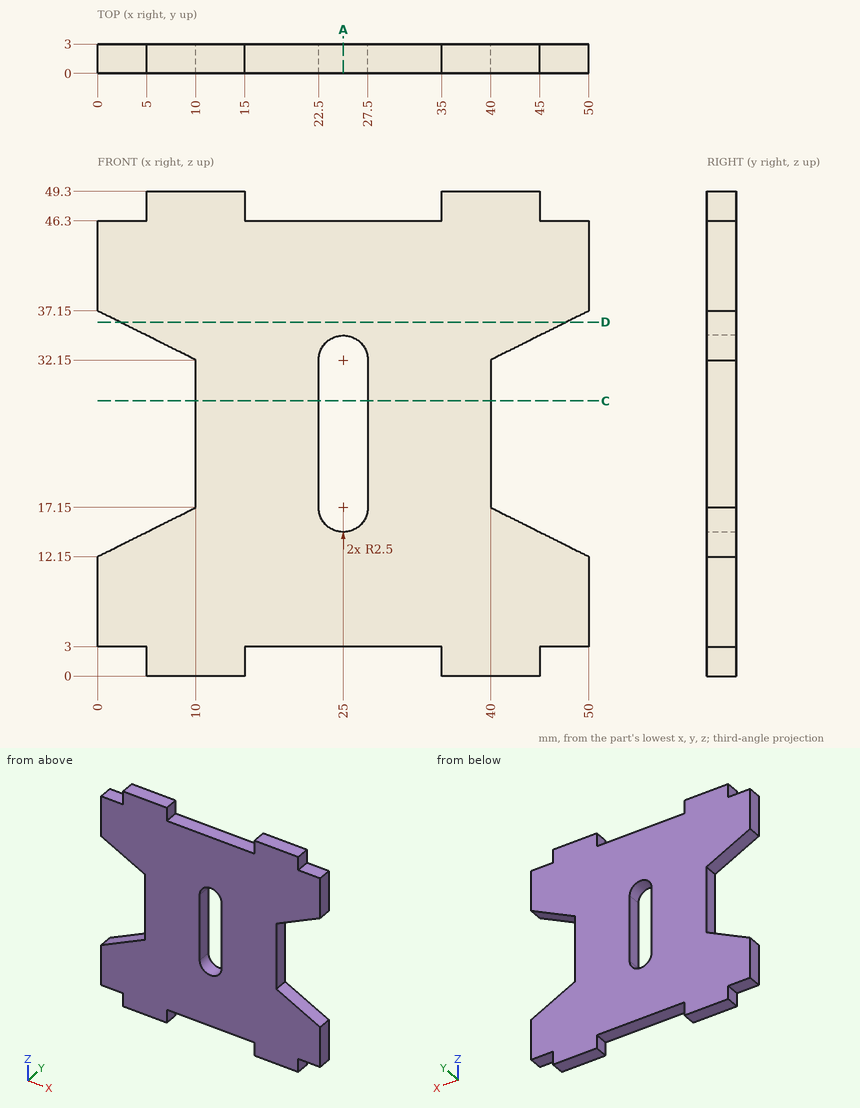
Drawing for the job (mm, zero at the part's lowest x, y, z). Coordinates: 2 decimals unless noted, no trailing zeros. Loops run counter-clockwise (first coordinate to the right, second up) from the corner with the lowest first, then second, coordinate; pieces in that order, holes last. Notation, with made-up numbers: (-9.5, 2.5) - (27.5, 2.5) arc R19 ccw to (27.5, 26.5) - close; hole circle Ø3 at (12, 84.5). An arc over 180 degrees is marked (long way). Use CSV: the item, a comma, the result in double quotes. Start each with the question number.
Q1. Cut at D-D, the plane z = 36. List the corners of the cut face in (x, y), then the cut area to 3 significant figures.
Q2. Probe probe 1 along X at (y, z) = (0.35, 27); probe 2 along Z at (x, y) = (29, 1.5); probe 3 along Z at (x, y) = (2.5, 1.5). List the from-to ranges inside material, lowest first. Write a range as from..to.
Q3. Cut at A-A, the plane x = 25. List the corners of the cut face in (y, z), then the cut area to 3 significant figures.
Q4. Drop flat-ended pins along their axis: P1, Ø0.9, axis at x = 2, y = 1, coming from the -Z side; P2, Ø1.5, axis at y = 2, z = 28, coming from the -X side; P3, Ø0.9, axis at y = 1.5, z = 2, coming from the -X side. Give the stop position or say it passes through.
Q5. Cut at C-C, the plane z = 28. List the corners of the cut face in (x, y), then the cut area to 3 significant figures.
Here are the results:
1,outline,"(2.3, 0) - (47.7, 0) - (47.7, 3) - (2.3, 3) - close"
1,area,"136 mm2"
2,probe 1,"10..22.5, 27.5..40"
2,probe 2,"3..46.3"
2,probe 3,"3..13.4, 35.9..46.3"
3,outline,"(0, 3) - (3, 3) - (3, 14.65) - (0, 14.65) - close; (0, 34.65) - (3, 34.65) - (3, 46.3) - (0, 46.3) - close"
3,area,"69.9 mm2"
4,P1,"z = 3"
4,P2,"x = 10"
4,P3,"x = 5"
5,outline,"(10, 0) - (22.5, 0) - (22.5, 3) - (10, 3) - close; (27.5, 0) - (40, 0) - (40, 3) - (27.5, 3) - close"
5,area,"75.0 mm2"
